from build123d import *

# Parameters (mm, degrees)
SKETCH1_R           = 4
BOSS_EXTRUDE1_DEPTH = 9.525


with BuildPart() as part:
    # Sketch1 → Boss-Extrude1 (new body)
    with BuildSketch(Plane(origin=(0, 0, 0), x_dir=(1, 0, 0), z_dir=(0, 1, 0))):
        with BuildLine():
            Line((-6, 0), (0, 0))
            Line((0, 0), (6, 0))
            Line((6, 0), (6, -3.175))
            Line((6, -3.175), (14, -3.175))
            Line((14, -3.175), (14, 11.825))
            ThreePointArc((14, 11.825), (0, 25.825), (-14, 11.825))
            Line((-14, 11.825), (-14, 0))
            Line((-14, 0), (-6, -3.175))
            Line((-6, -3.175), (-6, 0))
        make_face()
        with Locations((0, 11.825)):
            Circle(SKETCH1_R, mode=Mode.SUBTRACT)
    extrude(amount=BOSS_EXTRUDE1_DEPTH)


solid = part.part
The listing builds one solid part. Answer for the finished solid, in the listing's coordinates (mm). A direction names the side the tool comes from. Give positions to 0.01 mm unless a question says otherwise; leave off trailing zeros. Order: outer loops, then holes, each group sorted by start corner. A loop starts at its lowest first (then second) coordinate and runs counter-clockwise, first axis right, second up. Notation, with made-up numbers: (31.5, 76.5) -> (61.5, 76.5) arc R31 cw to (61.5, 115.5) -> close; hole circle Ø7 at (25.5, 15). An arc over 180 degrees is marked (long way). Put each result on its own line as item: value.
Item 1: A cutting plane is placed at A-A on x = 0. Give the vertices of the cut face in (y, z) (3 decimals), plus the area to 3 significant figures.
Established:
outline: (0, -25.825) -> (9.525, -25.825) -> (9.525, -15.825) -> (0, -15.825) -> close; (0, -7.825) -> (9.525, -7.825) -> (9.525, 0) -> (0, 0) -> close
area: 170 mm^2
Item 2: A cutting plane is placed at B-B on y = 1. Give the vertices of the cut face in (x, z) (3 decimals), plus the area to 3 significant figures.
Established:
outline: (-14, -11.825) arc R14 ccw to (14, -11.825) -> (14, 3.175) -> (6, 3.175) -> (6, 0) -> (-6, 0) -> (-6, 3.175) -> (-14, 0) -> close; hole circle Ø8 at (0, -11.825)
area: 627 mm^2
Item 3: Given P1, Ø5, axis at x = -3, y = 8, coming from the -Z side; P2, Ø4, axis at x = 3.5, y = 2, coming from the +Z side, each flat-ended and moving along its own axis, determine where each tip first touches the part or whether it passes through.
Established:
P1: stops at z = -25.82
P2: stops at z = 0
Item 4: For a pull along Z with two mould halves and no side action, classify faces 1 (the face through (10, 5, 3.175)), 2 (the face through (-0.87, 4.7, -7.92)), 3 (the face through (14, 5, -4)) as released by +Z, released by -Z, zero draft, split by the parting line, or undercut.
Established:
face 1: released by +Z
face 2: undercut
face 3: zero draft
Item 5: Straight lines are drawn through the part: line 1 (Z direction, x = 0, y = 6) (3 decimals); line 2 (Z direction, x = -2.5, y = 3.5); line 3 (X direction, y = 5, z = -8.25). For each, find the intervals that lie inside material, in ascending order.
Established:
line 1: z = -25.825 to -15.825, -7.825 to 0
line 2: z = -25.6 to -14.95, -8.7 to 0
line 3: x = -14 to -1.79, 1.79 to 14
Item 6: For faces 4 (the face through (3, 9.525, -8)), 5 (the face through (6, 5, 2)), determine the directions among +Z, -Z, +X, -X, +Y, -Y from which every point of the face is accessible in a straight line to the end or side of a thin tool.
Established:
face 4: +Z, -Z, +X, -X, +Y
face 5: +Z, +Y, -Y
Item 7: A cutting plane is placed at D-D on z = -20. Give the vertices of the cut face in (x, y) (3 decimals).
Established:
outline: (-11.365, 0) -> (11.365, 0) -> (11.365, 9.525) -> (-11.365, 9.525) -> close
Item 8: A cutting plane is placed at C-C on x = 12. Give the vertices of the cut face in (y, z) (3 decimals), plus the area to 3 significant figures.
Established:
outline: (0, -19.036) -> (9.525, -19.036) -> (9.525, 3.175) -> (0, 3.175) -> close
area: 212 mm^2
